Part print with two shaded views. Sizes in mm from the minimum x, y, z corner. Coordinates: 2 decimals unless noted, no trailing zeros. Loops run counter-clockwise (first coordinate to the right, second up) from the corner with the lowest first, then second, coordinate; pieces in that order, holes last.
(1) Wall check: L1, parallel to X at y = 42.5, z = 3.1; L2, parallel to X at y = 42.5, z = 8.3. Give the ranges that are in metal, low to high.
(2) Slice it at C-C (z = 3.75). Give the cut face in (x, y), and give its area (3 significant figures).
(3) Slice it at A-A (x = 42.5). Give the cut face in (y, z).
(4) Slice it at B-B (y = 72.5). Give the cut face in (x, z), and give its area (3 significant figures).
(5) Flat gauge pins, fed straight in: P1, Ø8, axis at x = 12.5, y = 42.5, coming from the -Z side; P2, Ø14.5, axis at x = 42.5, y = 12.5, coming from the +Z side. Where does each tip first touch, or does it go through?
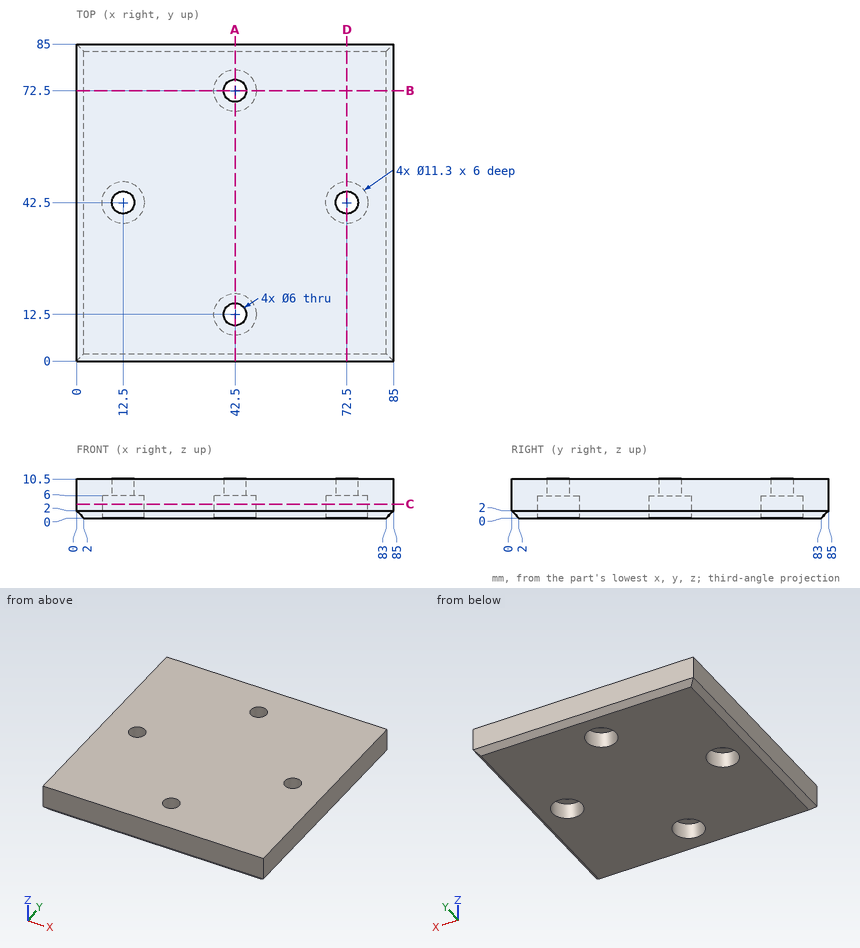
Response values:
1. L1: x = 0 to 6.85, 18.15 to 66.85, 78.15 to 85
1. L2: x = 0 to 9.5, 15.5 to 69.5, 75.5 to 85
2. outline: (0, 0) - (85, 0) - (85, 85) - (0, 85) - close; hole circle Ø11.3 at (12.5, 42.5); hole circle Ø11.3 at (42.5, 12.5); hole circle Ø11.3 at (42.5, 72.5); hole circle Ø11.3 at (72.5, 42.5)
2. area: 6,820 mm2
3. outline: (0, 2) - (2, 0) - (6.85, 0) - (6.85, 6) - (9.5, 6) - (9.5, 10.5) - (0, 10.5) - close; (15.5, 6) - (18.15, 6) - (18.15, 0) - (66.85, 0) - (66.85, 6) - (69.5, 6) - (69.5, 10.5) - (15.5, 10.5) - close; (75.5, 6) - (78.15, 6) - (78.15, 0) - (83, 0) - (85, 2) - (85, 10.5) - (75.5, 10.5) - close
4. outline: (0, 2) - (2, 0) - (36.85, 0) - (36.85, 6) - (39.5, 6) - (39.5, 10.5) - (0, 10.5) - close; (45.5, 6) - (48.15, 6) - (48.15, 0) - (83, 0) - (85, 2) - (85, 10.5) - (45.5, 10.5) - close
4. area: 794 mm2
5. P1: stops at z = 6
5. P2: stops at z = 10.5
